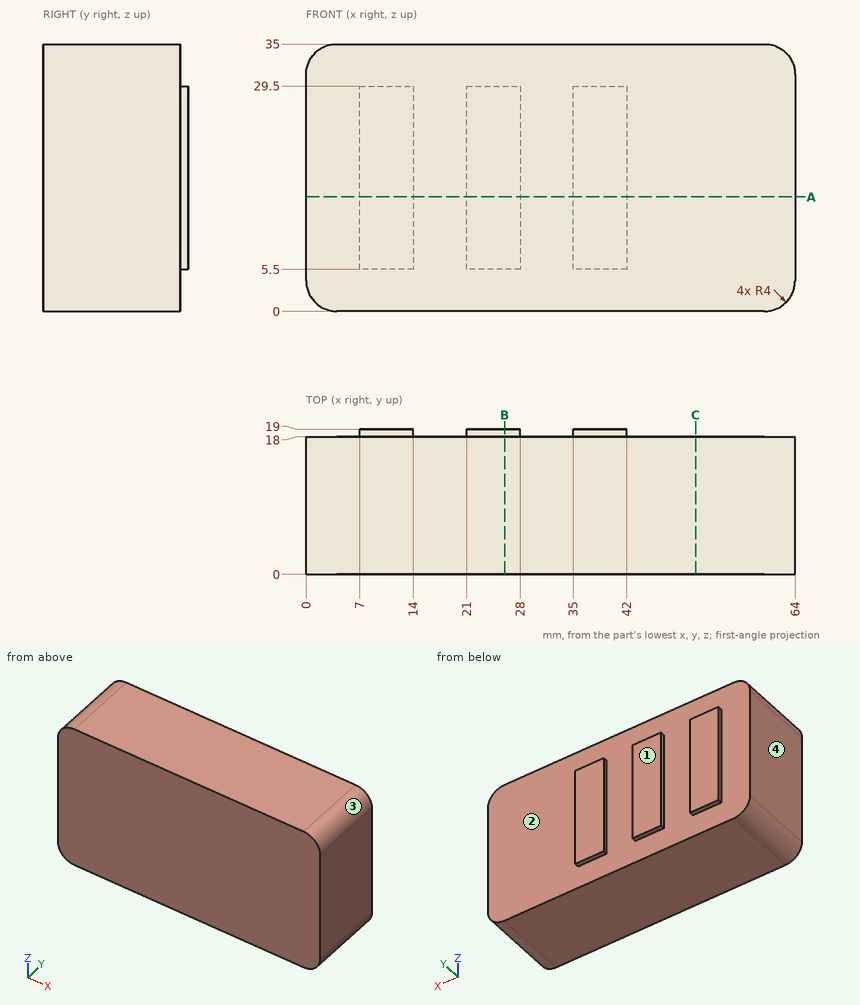
Input: dimensioned drawing with shaded views. Units: mm. Origin: part minimum x, y, z. Give positions to 0.01 mm unless a question says otherwise; leave off trailing zeros. Loops run counter-clockwise (first coordinate to the right, second up) from the corner with the lowest first, then second, coordinate; pieces in that order, holes last. Notation, with made-up numbers: M 14.25,34 L 54.25,34 A8 ccw 54.25,49 Z; hole C 83.5,-40 d4. An arc over 180 degrees is marked long. Put each result on its own line as item: value.
1) First-contact query: P1, Ø0.5, axis at x = 11.5, y = 18.5, coming from the +Z side; P2, Ø0.8, axis at x = 25.5, y = 18.5, coming from the -Z side; P3, Ø0.5, axis at y = 18.5, z = 22, coming from the -X side. Flat tips, straight axial feed; report the tip coordinate or a pass-through.
Computed values:
P1: stops at z = 29.5
P2: stops at z = 5.5
P3: stops at x = 7
2) Cut plane A-A, the plane z = 15. Return the cut outline in (x, y), plus the area to 3 significant figures.
Computed values:
outline: M 0,0 L 64,0 L 64,18 L 42,18 L 42,19 L 35,19 L 35,18 L 28,18 L 28,19 L 21,19 L 21,18 L 14,18 L 14,19 L 7,19 L 7,18 L 0,18 Z
area: 1,170 mm^2
3) Material intervals for L1, parallel to Y at x = 33, z = 5; L2, parallel to X at y = 10, z = 3.5; L3, parallel to X at y = 11.5, z = 2, sorted ascending. Write a range as from..to.
Computed values:
L1: y = 0..18
L2: x = 0.03..63.97
L3: x = 0.54..63.46
4) Mould query, pull axis X, two halves, no side actions, for the marked faces 1, 2, 3 and 4. Classes: released by +X, released by -X, zero draft, split by the parting line, or undercut.
Computed values:
face 1: zero draft
face 2: undercut
face 3: released by +X
face 4: released by -X
5) Cut plane C-C, the plane x = 51. Return the cut outline in (y, z), plus the area to 3 significant figures.
Computed values:
outline: M 0,0 L 18,0 L 18,35 L 0,35 Z
area: 630 mm^2
6) Cut plane B-B, the plane x = 26. Return the cut outline in (y, z).
Computed values:
outline: M 0,0 L 18,0 L 18,5.5 L 19,5.5 L 19,29.5 L 18,29.5 L 18,35 L 0,35 Z
